Autodesk Inventor part; units mm, degrees
ref_plane "YZ Plane" through (0, 0, 0) normal (1, 0, 0) x (0, 1, 0)
ref_plane "XZ Plane" through (0, 0, 0) normal (0, 1, 0) x (-1, 0, 0)
ref_plane "XY Plane" through (0, 0, 0) normal (0, 0, 1) x (1, 0, 0)
sketch "Boceto1" plane through (0, 0, 0) normal (0, 0, 1) x (1, 0, 0)
  circle A0 centre (0, 0) radius 50
  dimension "d0" = 100
extrude "Extrusión1" add sketch "Boceto1" along normal blind 3.2
sketch "Boceto2" plane through (0, 0, 3.2) normal (0, 0, 1) x (1, 0, 0)
  circle A0 centre (-22, -11.99) radius 1.25
  circle A1 centre (-22, -29.99) radius 1.25
  circle A2 centre (22, -29.99) radius 1.25
  circle A3 centre (22, -11.99) radius 1.25
  line L0 (-29, 1.01) -> (-59, 1.01)
  line L1 (-59, 1.01) -> (-59, -41.99)
  line L2 (-59, -41.99) -> (-29, -41.99)
  line L3 (-29, -41.99) -> (-29, 1.01)
  line L4 (29, 1.01) -> (59, 1.01)
  line L5 (59, 1.01) -> (59, -41.99)
  line L6 (59, -41.99) -> (29, -41.99)
  line L7 (29, -41.99) -> (29, 1.01)
  circle A4 centre (0, 0) radius 4.16 construction
  line L8 (-4.16, 4.16) -> (4.16, 4.16) construction
  line L9 (4.16, 4.16) -> (4.16, -11.99) construction
  line L10 (4.16, -11.99) -> (-4.16, -11.99) construction
  line L11 (-4.16, -11.99) -> (-4.16, 4.16) construction
  dimension "d3" = 2.5
  dimension "d4" = 44
  dimension "d5" = 22
  dimension "d6" = 18
  dimension "d7" = 43
  dimension "d8" = 30
  dimension "d9" = 12
  dimension "d10" = 7
  dimension "d11" = 7
  dimension "d12" = 8.32
  dimension "d13" = 16.15
extrude "Extrusión2" cut sketch "Boceto2" against normal through all
sketch "Boceto3" plane through (0, 0, 3.2) normal (0, 0, 1) x (1, 0, 0)
  circle A0 centre (-7.83, 42) radius 1.25
  circle A1 centre (7.83, 42) radius 1.25
  arc A2 (49.9898, 1.01) -> (-49.9898, 1.01) centre (0, 0) ccw
  dimension "d16" = 15.66
  dimension "d17" = 2.5
  dimension "d18" = 7.83
  dimension "d19" = 42
extrude "Extrusión3" cut sketch "Boceto3" against normal through all
sketch "Boceto4" plane through (0, 0, 3.2) normal (0, 0, 1) x (1, 0, 0)
  line L0 (-16.5, -9.49) -> (-10.5, -9.49)
  line L1 (-10.5, -9.49) -> (-10.5, -15.49)
  line L2 (-10.5, -15.49) -> (-16.5, -15.49)
  line L3 (-16.5, -15.49) -> (-16.5, -9.49)
  line L4 (10.5, -9.49) -> (16.5, -9.49)
  line L5 (16.5, -9.49) -> (16.5, -15.49)
  line L6 (16.5, -15.49) -> (10.5, -15.49)
  line L7 (10.5, -15.49) -> (10.5, -9.49)
  circle A0 centre (-22, -11.99) radius 1.25
  circle A1 centre (22, -11.99) radius 1.25
  line L8 (-16.5, -26.49) -> (-10.5, -26.49)
  line L9 (-10.5, -26.49) -> (-10.5, -32.49)
  line L10 (-10.5, -32.49) -> (-16.5, -32.49)
  line L11 (-16.5, -32.49) -> (-16.5, -26.49)
  line L12 (10.5, -26.49) -> (16.5, -26.49)
  line L13 (16.5, -26.49) -> (16.5, -32.49)
  line L14 (16.5, -32.49) -> (10.5, -32.49)
  line L15 (10.5, -32.49) -> (10.5, -26.49)
  circle A2 centre (-22, -29.99) radius 1.25
  point P0 (0, 0)
  dimension "d22" = 6
  dimension "d23" = 5.5
  dimension "d24" = 5.5
  dimension "d25" = 2.5
  dimension "d26" = 6
  dimension "d27" = 6
  dimension "d28" = 6
  dimension "d32" = 2.5
extrude "Extrusión4" cut sketch "Boceto4" against normal through all contours L0 L1 L2 L3 | L4 L5 L6 L7 | L8 L9 L10 L11 | L12 L13 L14 L15
sketch "Boceto5" plane through (0, 0, 3.2) normal (0, 0, 1) x (1, 0, 0)
  circle A0 centre (0, -44) radius 1.75
  arc A1 (49.9898, 1.01) -> (-49.9898, 1.01) centre (0, 0) ccw
  circle A2 centre (-37.5, 20.9519) radius 1.75
  circle A3 centre (37.5, 20.9519) radius 1.75
  point P0 (-27.1448, -41.99)
  point P1 (27.1448, -41.99)
  dimension "d33" = 3.5
  dimension "d34" = 44
  dimension "d35" = 37.5
  dimension "d36" = 37.5
  dimension "d37" = 75
extrude "Extrusión5" cut sketch "Boceto5" against normal through all
sketch "Boceto6" plane through (0, 0, 3.2) normal (0, 0, 1) x (1, 0, 0)
  circle A0 centre (0, 0) radius 1
  dimension "d41" = 2
extrude "Extrusión6" cut sketch "Boceto6" against normal through all
sketch "Boceto7" plane through (0, 0, 3.2) normal (0, 0, 1) x (1, 0, 0)
  circle A0 centre (0, 0) radius 1
  line L0 (0, 0) -> (-40, -20.99)
  line L1 (-16.5, -26.49) -> (-10.5, -26.49)
  line L2 (-10.5, -15.49) -> (-16.5, -15.49)
  line L3 (-29, 1.01) -> (-29, -40.7308)
  line L4 (0, 0) -> (40, -20.99)
  line L5 (29, -40.7308) -> (29, 1.01)
  line L6 (0, 0) -> (0, -20.99)
  dimension "d44" = 11
  dimension "d45" = 5.5
  dimension "d46" = 11
  dimension "d47" = 45.1728
  dimension "d48" = 11
  dimension "d49" = 45.1728
  dimension "d50" = 80
  dimension "d51" = 20.99
equation "\"d37\" = 2 * d35"
properties part number "Base"
Part model, mm, in its own coordinate system. Coordinates: 2 decimals unless noted, no trailing zeros. Write each loop counter-clockwise with the first axis right and the second up, starting at its lowest first coordinate (ties: lowest second). Pieces come first, ordered by that corner, then holes.
Item 1: Slice it at B-B (y = 42). Write the cut outline in (x, z).
Item 2: Slice it at A-A (x = 37.5). Write the cut outline in (y, z), and give its area (3 significant figures).
Item 3: Mould opens along Y. For faces 1 (the face through (-1, 12, 3.2)), 2 (the face through (0, -50, 2)), 3 (the face through (-16.5, -30, 2)), 4 (the face through (-1.09, 49.99, 1.58)) say: released by +Y, released by -Y, zero draft, split by the parting line, or undercut.
Item 4: Slice it at D-D (y = -44). Write the cut outline in (x, z), and give its area (3 significant figures).
Item 5: Pin check, flat tips, straight feed: pin 1 (1 mm diameter, centred on y = -29, z = 1.5, fed in from -X); pin 2 (1 mm diameter, centred on x = 13, z = 2, fed in from +Y); pin 3 (2 mm diameter, centred on x = 22, y = -11.99, fed in from +Z); pin 4 (4 mm diameter, centred on x = 22, y = -29.99, fed in from +Z). Stop position of each tip, or through.
Item 6: Probe line 1 (X direction, y = -28, z = 1.2); line 2 (Y direction, x = 0, z = 1.45); line 3 (X direction, y = 43, z = 0.3). List the from-to ranges inside material, lowest first.
Item 7: Slice it at C-C (x = 22). Write the cut outline in (y, z).
Results found:
1. outline: (-27.13, 0) - (-9.08, 0) - (-9.08, 3.2) - (-27.13, 3.2) - close; (-6.58, 0) - (6.58, 0) - (6.58, 3.2) - (-6.58, 3.2) - close; (9.08, 0) - (27.13, 0) - (27.13, 3.2) - (9.08, 3.2) - close
2. outline: (1.01, 0) - (19.2, 0) - (19.2, 3.2) - (1.01, 3.2) - close; (22.7, 0) - (33.07, 0) - (33.07, 3.2) - (22.7, 3.2) - close
2. area: 91.4 mm2
3. face 1: zero draft
3. face 2: released by -Y
3. face 3: undercut
3. face 4: released by +Y
4. outline: (-23.75, 0) - (-1.75, 0) - (-1.75, 3.2) - (-23.75, 3.2) - close; (1.75, 0) - (23.75, 0) - (23.75, 3.2) - (1.75, 3.2) - close
4. area: 141 mm2
5. pin 1: stops at x = -29
5. pin 2: stops at y = 48.41
5. pin 3: passes through
5. pin 4: stops at z = 3.2
6. line 1: x = -29 to -16.5, -10.5 to 10.5, 16.5 to 29
6. line 2: y = -50 to -45.75, -42.25 to -1, 1 to 50
6. line 3: x = -25.51 to -8.58, -7.08 to 7.08, 8.58 to 25.51
7. outline: (-44.9, 0) - (-31.24, 0) - (-31.24, 3.2) - (-44.9, 3.2) - close; (-28.74, 0) - (-13.24, 0) - (-13.24, 3.2) - (-28.74, 3.2) - close; (-10.74, 0) - (44.9, 0) - (44.9, 3.2) - (-10.74, 3.2) - close
